from build123d import *

# Parameters (mm, degrees)
SKETCH1_R               = 29.999999999999996
BOSS_EXTRUDE1_DEPTH     = 60
CUT_EXTRUDE2_DEPTH      = 60
CUT_EXTRUDE2_DEPTH_BACK = 60
CUT_EXTRUDE6_DEPTH      = 60
CUT_EXTRUDE6_DEPTH_BACK = 60
CUT_EXTRUDE7_DEPTH      = 0.0001
BOSS_EXTRUDE2_DEPTH     = 0.0001


with BuildPart() as part:
    # Sketch1 → Boss-Extrude1 (new body)
    with BuildSketch(Plane.XY):
        Circle(SKETCH1_R)
    extrude(amount=BOSS_EXTRUDE1_DEPTH)

    # Sketch2 → Cut-Extrude2 (cut, two sides: drawn at the far end of the back side and taken through both)
    with BuildSketch(Plane(origin=(0, 0, 0), x_dir=(1, 0, 0), z_dir=(0, 1, 0)).offset(-CUT_EXTRUDE2_DEPTH_BACK)):
        with BuildLine():
            Line((-7.1054e-13, 0), (-30, 0))
            Line((-30, 0), (-30, -30.00000000000002))
            ThreePointArc((-30, -29.999999999999996), (-21.213203435596675, -8.786796564403826), (-7.1093e-13, 0))
        make_face()
        with BuildLine():
            ThreePointArc((2.2327e-12, -60), (-21.213203435595638, -51.21320343559721), (-30, -29.999999999999996))
            Line((-30, -30.00000000000002), (-30, -60))
            Line((-30, -60), (2.2311e-12, -60))
        make_face()
        with BuildLine():
            Line((30, -60), (30, -30))
            ThreePointArc((30, -30.000000000000007), (21.21320343559721, -51.21320343559564), (2.2327e-12, -60))
            Line((2.2311e-12, -60), (30, -60))
        make_face()
        with BuildLine():
            Line((30, 0), (-7.1054e-13, 0))
            ThreePointArc((-7.1093e-13, 0), (21.213203435596174, -8.786796564403325), (30, -30))
            Line((30, -30), (30, 0))
        make_face()
    extrude(amount=CUT_EXTRUDE2_DEPTH + CUT_EXTRUDE2_DEPTH_BACK, mode=Mode.SUBTRACT)

    # Sketch7 → Cut-Extrude6 (cut, two sides: drawn at the far end of the back side and taken through both)
    with BuildSketch(Plane(origin=(0, 0, 0), x_dir=(0, 0, -1), z_dir=(1, 0, 0)).offset(-CUT_EXTRUDE6_DEPTH_BACK)):
        Polygon((0, 30), (-60, -30), (-60, 30), align=None)
    extrude(amount=CUT_EXTRUDE6_DEPTH + CUT_EXTRUDE6_DEPTH_BACK, mode=Mode.SUBTRACT)

    # Sketch8 → Cut-Extrude7 (cut)
    with BuildSketch(Plane(origin=(0, 15.000000000000005, 15.000000000000004), x_dir=(1, 0, 0), z_dir=(0, 0.7071067811865477, 0.7071067811865475))):
        with BuildLine():
            ThreePointArc((21.21320343559647, 3.5988e-13), (14.999999999999906, 15.000000000000137), (4.43e-15, 21.21320343559642))
            Line((0, 21.21320343559642), (3.068e-14, 8.78679656440357))
            ThreePointArc((3.068e-14, 8.78679656440357), (11.480502970952555, 6.50318253974223), (21.213203435596192, 2.2737e-13))
        make_face()
        with BuildLine():
            ThreePointArc((21.213203435596192, 2.2737e-13), (11.480502970952555, 6.50318253974223), (3.068e-14, 8.78679656440357))
            Line((3.068e-14, 8.78679656440357), (1.0474e-13, -21.213203435596412))
            ThreePointArc((1.0474e-13, -21.213203435596412), (15.000000000000192, -14.999999999999844), (21.21320343559647, 3.6459e-13))
        make_face()
        with BuildLine():
            add(Edge.make_bspline(
                [(30, -21.21320343559644), (30.000000000000018, 21.213203435596398), (1.677e-14, 21.21320343559642)],
                knots=[4.71238898038469, 4.71238898038469, 4.71238898038469, 6.283185307179586, 6.283185307179586, 6.283185307179586], degree=2, weights=[1, 0.7071067811865476, 1]))
            ThreePointArc((4.43e-15, 21.21320343559642), (14.999999999999906, 15.000000000000137), (21.21320343559647, 3.5988e-13))
            ThreePointArc((21.213203435596192, 2.2737e-13), (27.71638597533854, -9.732700464643589), (29.999999999999996, -21.21320343559643))
        make_face()
        with BuildLine():
            ThreePointArc((29.999999999999996, -21.21320343559643), (27.71638597533854, -9.732700464643589), (21.213203435596192, 2.2737e-13))
            ThreePointArc((21.21320343559647, 3.6459e-13), (15.000000000000192, -14.999999999999844), (1.0474e-13, -21.213203435596412))
            Line((1.0474e-13, -21.213203435596412), (29.999999999999996, -21.213203435596427))
        make_face()
    extrude(amount=-CUT_EXTRUDE7_DEPTH, mode=Mode.SUBTRACT)

    # Sketch9 → Boss-Extrude2 (add)
    with BuildSketch(Plane(origin=(0, 15.000000000000005, 15.000000000000004), x_dir=(1, 0, 0), z_dir=(0, 0.7071067811865477, 0.7071067811865475))):
        with BuildLine():
            ThreePointArc((29.99999999995833, -21.213203435596427), (21.21320343556702, -42.42640687116332), (1.7636e-13, -51.213203435554746))
            Line((1.691e-13, -51.213203435554746), (1.9602e-13, -63.639610306789265))
            add(Edge.make_bspline(
                [(-1.309e-14, -63.63961030678927), (29.999999999999982, -63.63961030678929), (30, -21.21320343559644)],
                knots=[3.141592653589793, 3.141592653589793, 3.141592653589793, 4.71238898038469, 4.71238898038469, 4.71238898038469], degree=2, weights=[1, 0.7071067811865476, 1]))
        make_face()
        with BuildLine():
            Line((29.99999999995833, -21.213203435596427), (1.0408e-13, -21.213203435596416))
            Line((1.0408e-13, -21.213203435596416), (1.691e-13, -51.213203435554746))
            ThreePointArc((1.7636e-13, -51.213203435554746), (21.21320343556702, -42.42640687116332), (29.99999999995833, -21.213203435596427))
        make_face()
    extrude(amount=BOSS_EXTRUDE2_DEPTH)


solid = part.part
Could you check a few things on this model? Use its own coordinates, in mm. Round coordinates to 2 decimals unless told otherwise and drop trailing zeros. Write each loop counter-clockwise with the first axis right and the second up, starting at its lowest first coordinate (ties: lowest second). Pieces come first, ordered by that corner, then holes. Notation, with made-up numbers: (52, -21) -> (98, -21) arc R15 cw to (98, 6) -> close; hole circle Ø6 at (41, 62). An arc over 180 degrees is marked (long way). Use a Markdown table: item, result.
1. Please list where these lines run through material, in increasing order: probe 1 along Y at (x, z) = (-27.5, 31); probe 2 along X at (y, z) = (-9.5, 5.5); probe 3 along Z at (x, y) = (4, 1.5).
Answer key:
| item | result |
|---|---|
| probe 1 | y = -11.99 to -1 |
| probe 2 | x = -17.31 to 17.31 |
| probe 3 | z = 0.27 to 28.5 |
2. If we section it at B-B (x = -12.5): List the corners of the cut face in (y, z) for me.
Answer key:
| item | result |
|---|---|
| outline | (-27.27, 2.73) -> (27.27, 2.73) -> (-27.27, 57.27) -> close |
3. For pin 1 Ø4 at (x, z) = (1.5, 33.5) entering from -Y; pin 2 Ø3 at (x, y) = (-1, -0.5) entering from +Z; pin 3 Ø2 at (x, y) = (7.5, -10.5) entering from -Z; pin 4 Ø1 at (x, z) = (19.5, 49) entering from +Y, each with a flat end and sliding along its axis, tell me the tip position at first contact or that it passes through.
Answer key:
| item | result |
|---|---|
| pin 1 | stops at y = -30 |
| pin 2 | stops at z = 32 |
| pin 3 | stops at z = 0.71 |
| pin 4 | stops at y = -18.5 |
